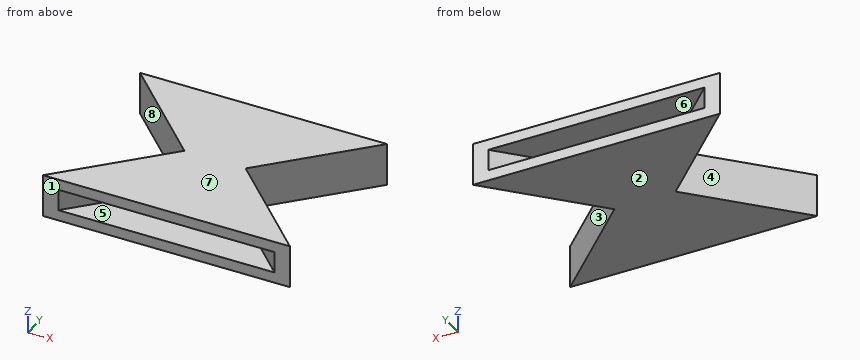
from build123d import *

# Parameters (mm, degrees)
F1_DEPTH = 14
F2_T     = -3.5


with BuildPart() as f1:
    # F0 (on Top) → F1 (new body)
    with BuildSketch(Plane.XY):
        Polygon((39.8995, 30), (-39.8995, 30), (-9.8995, 0), (-39.8995, -30), (39.8995, -30), (9.8995, 0), align=None)
    extrude(amount=F1_DEPTH)

    # F2
    f2_openings = [f1.faces().sort_by_distance(p)[0] for p in [
        (0, -30, 7),
        (0, 30, 7),
    ]]
    offset(amount=F2_T, openings=f2_openings, kind=Kind.INTERSECTION)


solid = f1.part
Model file for the job. Use its own axes, mm. Face numbers are marked on the shaded views. A direction names the side the tool comes from. Coordinates: 2 decimals unless noted, no trailing zeros. Order: outer loops, then holes, each group sorted by start corner. A loop starts at its lowest first (then second) coordinate and runs counter-clockwise, first axis right, second up. Notation, with made-up numbers: M 73,18.5 L 116,18.5 A20 cw 116,23.5 Z; hole C -22.5,69.25 d4. An arc over 180 degrees is marked long. Return JSON: item names as keys, results as strings.
1. Saw through at C-C (x = -28). Give the cut face in (y, z).
Ans:
{"outline": "M -30,0 L -18.1,0 L -18.1,14 L -30,14 L -30,10.5 L -23.05,10.5 L -23.05,3.5 L -30,3.5 Z; M 18.1,0 L 30,0 L 30,3.5 L 23.05,3.5 L 23.05,10.5 L 30,10.5 L 30,14 L 18.1,14 Z"}
2. Saw through at A-A (z = 6.5). Give the cut face in (x, y), and give its area (3 significant figures).
Ans:
{"outline": "M -39.9,-30 L -34.95,-30 L -4.95,0 L -34.95,30 L -39.9,30 L -9.9,0 Z; M 4.95,0 L 34.95,-30 L 39.9,-30 L 9.9,0 L 39.9,30 L 34.95,30 Z", "area": "594 mm^2"}
3. Flat gauge pins, fed straight in: pin 1 (2 mm diameter, centred on y = 18.5, z = 3.5, fed in from +X); pin 2 (1.5 mm diameter, centred on x = 14.5, z = 7.5, fed in from -Y); pin 3 (8 mm diameter, centred on y = 17, z = 2, fed in from +X). Where does each tip first touch, or does it go through?
Ans:
{"pin 1": "x = 29.4", "pin 2": "y = -10.3", "pin 3": "x = 30.9"}
4. Pull direction Z, two halves, no side cores. Call the marked faces 6, 7 and 8: +Z half, -Z half, draft (parallel to the pull), parting line (faces both ways), or undercut.
Ans:
{"face 6": "undercut", "face 7": "+Z half", "face 8": "draft"}
5. Saw through at D-D (z = 12). Give the cut face in (x, y).
Ans:
{"outline": "M -39.9,-30 L 39.9,-30 L 9.9,0 L 39.9,30 L -39.9,30 L -9.9,0 Z"}
6. Tool access for the marked faces 1, 2, 3, 4 and 5: list every direction of +Z, -Z, +X, -X, +Y, -Y with a clear straight run to the whole face (end or side of a thin tool).
Ans:
{"face 1": "+Z, -Z, +X, -X, -Y", "face 2": "-Z, +X, -X, +Y, -Y", "face 3": "+Z, -Z, +X", "face 4": "+Z, -Z, -X", "face 5": "none"}
7. Saw through at B-B (y = 4). Give the cut face in (x, z), and give its area (3 significant figures).
Ans:
{"outline": "M -13.9,0 L 13.9,0 L 13.9,14 L -13.9,14 Z; hole M -8.95,3.5 L 8.95,3.5 L 8.95,10.5 L -8.95,10.5 Z", "area": "264 mm^2"}
8. Drill centre lines: probe 1 along Z at (x, y) = (-13, -17); probe 2 along Y at (x, z) = (34, 7.5); probe 3 along Y at (x, z) = (-20, 10). Where is each one in solid material? Low to high.
Ans:
{"probe 1": "0 to 3.5, 10.5 to 14", "probe 2": "-29.05 to -24.1, 24.1 to 29.05", "probe 3": "-15.05 to -10.1, 10.1 to 15.05"}
